Autodesk Inventor part; units mm, degrees
ref_plane "YZ Plane" through (0, 0, 0) normal (1, 0, 0) x (0, 1, 0)
ref_plane "XZ Plane" through (0, 0, 0) normal (0, 1, 0) x (-1, 0, 0)
ref_plane "XY Plane" through (0, 0, 0) normal (0, 0, 1) x (1, 0, 0)
sketch "Sketch1" plane through (0, 0, 0) normal (0, 0, 1) x (1, 0, 0)
  circle A0 centre (0, 0) radius 2.5
  dimension "d0" = 5
extrude "Extrusion1" add sketch "Sketch1" along normal blind 8
sketch "Sketch2" plane through (0, 0, 8) normal (0, 0, 1) x (1, 0, 0)
  circle A0 centre (1.3581, 0) radius 0.6166
  circle A1 centre (-1.4059, 0) radius 0.6367
  point P0 (0, 0)
extrude "Extrusion2" add sketch "Sketch2" along normal blind 15
fillet "Fillet1" radius 2 1 edges at (-2.5, 0, 0)
properties part number "5mm_led"
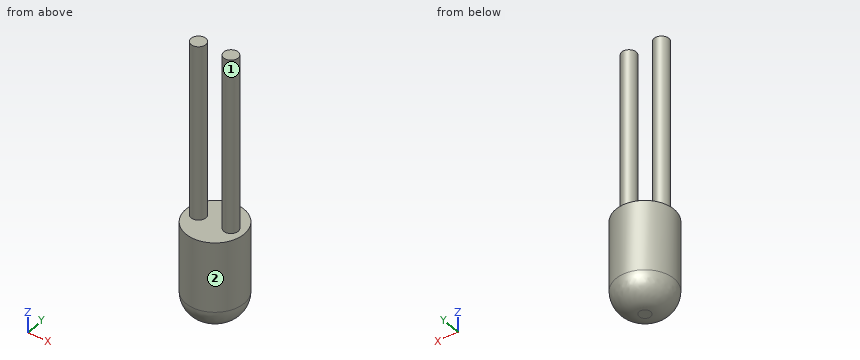
Check sheet for the modelled part. Datum: model origin and axes. Units: mm. Face numbers are marked on the shaded views. Give positions to 0.01 mm unless a question says otherwise; leave off trailing zeros. Order: outer loops, then holes, each group sorted by start corner. A loop starts at its lowest first (then second) coordinate and runs counter-clockwise, first axis right, second up. Notation, with made-up numbers: (83.5, 60.5) - (123.5, 60.5) arc R37 ccw to (123.5, 96.5) - close; hole circle Ø7 at (-26, 21). An arc over 180 degrees is marked (long way). Answer as CSV lines item,"result".
1. Section check A-A (z = 19). Record the boundary of the cut face in (x, y), then the cut area to 3 significant figures.
Result sheet:
outline,"circle Ø1.27 at (-1.41, 0); circle Ø1.23 at (1.36, 0)"
area,"2.47 mm²"
2. Go/stop test with flat-tipped pins: P1, Ø1.5, axis at x = 1, y = -1, coming from the -Z side; P2, Ø3, axis at y = 1.5, z = 3.5, coming from the -X side. Record where each tip stops, or that it passes through.
Result sheet:
P1,"z = 0.01"
P2,"x = -2.5"
3. Mould release check, pull along X, two halves, no side actions. Record for the marked faces 1 and 2: released by +X, released by -X, zero draft, split by the parting line, or undercut.
Result sheet:
face 1,"undercut"
face 2,"split by the parting line"
4. Scan lines: probe 1 along Z at (x, y) = (0.1, -0.4); probe 2 along X at (y, z) = (0.5, 10); probe 3 along X at (y, z) = (-0.4, 17.5). Record each from-to range of solid material in increasing order. Write a range as from..to.
Result sheet:
probe 1,"0..8"
probe 2,"-1.8..-1.01, 1..1.72"
probe 3,"-1.9..-0.91, 0.89..1.83"
